Input: part model. Units: mm. Frame: model coordinates. A direction names the side the tool comes from. Give positions to 0.01 mm unless a question says otherwise; leave off trailing zeros. Loops run counter-clockwise (first coordinate to the right, second up) from the corner with the lowest first, then second, coordinate; pieces in that order, holes last. Notation, with made-up numbers: (75.5, -32) -> (86.5, -32) arc R17 ccw to (86.5, -26) -> close; hole circle Ø4 at (49, -34). An arc over 180 degrees is marked (long way). One line per question, with ' | ' between items.
from build123d import *

# Parameters (mm, degrees)
F3_DEPTH      = 19.05
F3_DEPTH_BACK = 19.05
F4_R          = 12.7
F5_DEPTH      = 25.4
F8_DEPTH      = 69.851
F9_DEPTH      = 25.4


with BuildPart() as f1:
    # F0 (on Front) → F1 (revolve)
    with BuildSketch(Plane.XZ):
        Polygon((25.4, 0), (12.7, 0), (12.7, -63.5), (4.7625, -63.5), (4.7625, -69.85), (19.05, -69.85), (19.05, -6.444424), (25.4, -6.444424), align=None)
    revolve(axis=Axis((0, 0, -15.169185), (0, 0, 1)))


with BuildPart() as f3:
    # F2 (on Front) → F3 (new body, two sides)
    with BuildSketch(Plane.XZ) as f3_sk:
        Polygon((51.600001, 0), (0, 0), (-49.999999, 0), (-49.999999, -6.35), (0, -6.35), (51.600001, -6.35), align=None)
    extrude(amount=F3_DEPTH)
    extrude(f3_sk.sketch, amount=-F3_DEPTH_BACK)

    # F4 (on Top) → F5 (cut)
    with BuildSketch(Plane.XY):
        Circle(F4_R)
    extrude(amount=-F5_DEPTH, mode=Mode.SUBTRACT)

    # F6: union F1
    add(f1.part)

    # F7 (on Top) → F8 (cut, through all)
    with BuildSketch(Plane.XY):
        Polygon((0, -19.05), (-16.800521, -19.05), (-16.800521, -29.420776), (16.800521, -29.420776), (16.800521, -19.05), align=None)
        Polygon((-16.800521, 19.05), (0, 19.05), (16.800521, 19.05), (16.800521, 27.208871), (-16.800521, 27.208871), align=None)
    extrude(amount=-F8_DEPTH, mode=Mode.SUBTRACT)

    # F7 (on Top) → F9 (cut)
    with BuildSketch(Plane.XY):
        with BuildLine():
            Line((51.600001, -9.652), (51.600001, 9.652))
            Line((51.600001, 9.652), (35.052, 9.652))
            ThreePointArc((35.052, 9.652), (28.227005, 6.824995), (25.4, 0))
            ThreePointArc((25.4, 0), (28.227005, -6.824995), (35.052, -9.652))
            Line((35.052, -9.652), (51.600001, -9.652))
        make_face()
        with BuildLine():
            Line((-35.052, 9.652), (-49.999999, 9.652))
            Line((-49.999999, 9.652), (-49.999999, -9.652))
            Line((-49.999999, -9.652), (-35.052, -9.652))
            ThreePointArc((-35.052, -9.652), (-25.4, 0), (-35.052, 9.652))
        make_face()
    extrude(amount=-F9_DEPTH, mode=Mode.SUBTRACT)


solid = f3.part
1. Pull-direction query (Y, two-part tool) for faces 6 (the flat face through (5, 0, -63.5)), 7 (the cylindrical face through (-15.12, -11.59, -37.7)), 8 (the flat face through (-50, -14, -3)); classes: pulls with the +Y half, pulls with the -Y half, needs draft (parallel to the pull), parting line crosses it, or undercut.
Determined:
face 6: undercut | face 7: parting line crosses it | face 8: needs draft
2. Reachability of faces 1 (the cylindrical face through (-2.75, -12.4, -31.31)), 2 (the flat face through (-50, 14, -3)), 3 (the flat face through (43, -9.652, -3)), 4 (the flat face through (13, 0, 0)), 5 (the flat face through (-43, -9.652, -3)) from +Z, -Z, +X, -X, +Y, -Y: full face, straight path, thin tool, end or side. Return the list, or none.
Determined:
face 1: +Z | face 2: +Z, -Z, -X, +Y, -Y | face 3: +Z, -Z, +X | face 4: +Z, +X, -X, +Y, -Y | face 5: +Z, -Z, -X
3. Section query C-C (z = -26.5). Output: boundary loops of the cut face in (x, y).
Determined:
outline: circle Ø38.1 at (0, 0); hole circle Ø25.4 at (0, 0)
4. Section query B-B (y = 3.5). Output: boundary loops of the cut face in (x, z).
Determined:
outline: (-26.06, -6.35) -> (-25.16, -6.35) -> (-25.16, -6.44) -> (-18.73, -6.44) -> (-18.73, -69.85) -> (-3.23, -69.85) -> (-3.23, -63.5) -> (-12.21, -63.5) -> (-12.21, 0) -> (-26.06, 0) -> close; (3.23, -69.85) -> (18.73, -69.85) -> (18.73, -6.44) -> (25.16, -6.44) -> (25.16, -6.35) -> (26.06, -6.35) -> (26.06, 0) -> (12.21, 0) -> (12.21, -63.5) -> (3.23, -63.5) -> close
5. Section query A-A (x = -43.5). Output: boundary loops of the cut face in (y, z).
Determined:
outline: (-19.05, -6.35) -> (-9.65, -6.35) -> (-9.65, 0) -> (-19.05, 0) -> close; (9.65, -6.35) -> (19.05, -6.35) -> (19.05, 0) -> (9.65, 0) -> close
6. Ray query, line 1 along Y through (x, z) = (0, -67); line 2 along Y through (x, z) = (0, -45); line 3 along Z through (x, y) = (44, -11). Return the intervals inside material, ascending. Write a range as from..to.
Determined:
line 1: y = -19.05..-4.76, 4.76..19.05 | line 2: y = -19.05..-12.7, 12.7..19.05 | line 3: z = -6.35..0
7. Section query D-D (x = 8). Output: boundary loops of the cut face in (y, z).
Determined:
outline: (-19.05, -6.44) -> (-17.29, -6.44) -> (-17.29, -69.85) -> (17.29, -69.85) -> (17.29, -6.44) -> (19.05, -6.44) -> (19.05, 0) -> (9.86, 0) -> (9.86, -63.5) -> (-9.86, -63.5) -> (-9.86, 0) -> (-19.05, 0) -> close
8. Pin query (flat end, axial travel): P1, Ø5.5, axis at x = -30.5, y = -5.5, coming from the -Z side; P2, Ø21, axis at x = 30.5, y = 14, coming from the -Z side; P3, Ø1, axis at x = -39, y = -7.5, coming from the +Z side; P4, Ø3, axis at x = -13, z = -47, coming from the +Y side. Return the tip coordinate at first contact, or that it passes through.
Determined:
P1: stops at z = -6.35 | P2: stops at z = -6.44 | P3: passes through | P4: stops at y = 15.19
